Model file for the job. Use its own axes, mm. A direction names the side the tool comes from. Coordinates: 2 decimals unless noted, no trailing zeros. Write item = value, one per line. Start each with the question number.
from build123d import *

# Parameters (mm, degrees)
SKETCH1_W             = 20.25
SKETCH1_H             = 19.16
BOSS_EXTRUDE1_DEPTH   = 55.2
CUT_EXTRUDE2_DEPTH    = 60.572467634
CUT_EXTRUDE3_DEPTH    = 60.301443701
M6_TAPPED_HOLE1_D     = 5
M6_TAPPED_HOLE1_DEPTH = 15
M6_TAPPED_HOLE1_TIP   = 1.502151548


with BuildPart() as part:
    # Sketch1 → Boss-Extrude1 (new body)
    with BuildSketch(Plane(origin=(0, 0, 0), x_dir=(1, 0, 0), z_dir=(0, 1, 0))):
        Rectangle(SKETCH1_W, SKETCH1_H)
    extrude(amount=-BOSS_EXTRUDE1_DEPTH)

    # Sketch5 → Cut-Extrude2 (cut, through all)
    with BuildSketch(Plane(origin=(10.125, 0, 0), x_dir=(0, 0, -1), z_dir=(1, 0, 0))):
        Polygon((-9.58, -55.2), (0, -54.361858603), (9.58, -55.2), align=None)
    extrude(amount=-CUT_EXTRUDE2_DEPTH, mode=Mode.SUBTRACT)

    # Sketch6 → Cut-Extrude3 (cut, through all)
    with BuildSketch(Plane.XY.offset(9.58)):
        Polygon((-10.125, -55.2), (0, -54.361858603), (10.125, -55.2), align=None)
    extrude(amount=-CUT_EXTRUDE3_DEPTH, mode=Mode.SUBTRACT)

    # M6 Tapped Hole1
    with Locations(Plane(origin=(0, 0, 0), x_dir=(1, 0, 0), z_dir=(0, 1, 0))):
        with Locations((0, 0)):
            Hole(M6_TAPPED_HOLE1_D / 2, depth=M6_TAPPED_HOLE1_DEPTH)
            with Locations((0, 0, -(M6_TAPPED_HOLE1_DEPTH + M6_TAPPED_HOLE1_TIP / 2))):  # 118° drill point
                Cone(0, M6_TAPPED_HOLE1_D / 2, M6_TAPPED_HOLE1_TIP, mode=Mode.SUBTRACT)


solid = part.part
(1) Drop flat-ended pins along their axis: pin 1 Ø6 at (x, z) = (0, 0) entering from -Y; pin 2 Ø6 at (x, z) = (-2, -5.5) entering from +Y. Give the stop position or say it passes through.
(2) 3-axis set-ups, long thin cutter, end or side, ignore diameter. For faces 1 (the face through (-7.2, -54.6, 2.7)), 2 (the face through (0.54, -7.6, 2.44)), 3 (the face through (2.74, -54.59, -6.85)): which of +Z, -Z, +X, -X, +Y, -Y reach the whole face in a straight line?
(3) Mould opens along Z. For faces 4 (the face through (3.867, -54.682, 5.922)), 5 (the face through (0, -27, 9.58)), 6 (the face through (0, -27, -9.58)), 7 (the face through (6.258, -54.682, -3.658)) say: released by +Z, released by -Z, zero draft, split by the parting line, or undercut.
(4) Drill centre lines: line 1 along Z through (x, y) = (0, -9); line 2 along Y through (x, z) = (-6.25, -2.75); line 3 along Y through (x, z) = (-0.25, 4). Where is each one in solid material? Low to high.
Returned:
q1.pin_1 = -54.54
q1.pin_2 = 0
q2.face_1 = +X, -X, -Y
q2.face_2 = +Y
q2.face_3 = +Z, -Z, -Y
q3.face_4 = zero draft
q3.face_5 = released by +Z
q3.face_6 = released by -Z
q3.face_7 = undercut
q4.line_1 = -9.58 to -2.5, 2.5 to 9.58
q4.line_2 = -54.6 to 0
q4.line_3 = -54.38 to 0
